from build123d import *

# Parameters (mm, degrees)
SKETCH1_R                        = 4.826
BOSS_EXTRUDE1_DEPTH              = 6.35
F_18_0_1695_DIAMETER_HOLE1_D     = 4.3053
F_18_0_1695_DIAMETER_HOLE1_DEPTH = 25.4
F_18_0_1695_DIAMETER_HOLE1_TIP   = 1.293442612
SKETCH4_R                        = 6.2992
SKETCH4_R_2                      = 6.35
CUT_EXTRUDE1_DEPTH               = 3.175
SKETCH5_R                        = 6.2992
CUT_EXTRUDE2_DEPTH               = 3.175
F_17_64_0_26563_DIAMETER_HOLE1_D = 6.747002


with BuildPart() as part:
    # Sketch1 → Boss-Extrude1 (new body)
    with BuildSketch(Plane(origin=(0, 0, 0), x_dir=(1, 0, 0), z_dir=(0, 1, 0))):
        with BuildLine():
            Line((0, 12.7), (114.3, 12.7))
            ThreePointArc((114.3, 12.7), (127, 0), (114.3, -12.7))
            Line((114.3, -12.7), (0, -12.7))
            ThreePointArc((0, -12.7), (-12.7, 0), (0, 12.7))
        make_face()
        Circle(SKETCH1_R, mode=Mode.SUBTRACT)
    extrude(amount=BOSS_EXTRUDE1_DEPTH)

    # #18 (0.1695) Diameter Hole1
    with Locations(Plane(origin=(0, 6.35, 0), x_dir=(1, 0, 0), z_dir=(0, 1, 0))):
        with Locations((-9.652, 0), (4.826, 8.358877197), (4.826, -8.358877197)):
            Hole(F_18_0_1695_DIAMETER_HOLE1_D / 2, depth=F_18_0_1695_DIAMETER_HOLE1_DEPTH)
            with Locations((0, 0, -(F_18_0_1695_DIAMETER_HOLE1_DEPTH + F_18_0_1695_DIAMETER_HOLE1_TIP / 2))):  # 118° drill point
                Cone(0, F_18_0_1695_DIAMETER_HOLE1_D / 2, F_18_0_1695_DIAMETER_HOLE1_TIP, mode=Mode.SUBTRACT)

    # Sketch4 → Cut-Extrude1 (cut)
    with BuildSketch(Plane(origin=(0, 6.35, 0), x_dir=(1, 0, 0), z_dir=(0, 1, 0))):
        with Locations((76.2, 0)):
            Circle(SKETCH4_R)
        with Locations((114.3, 0)):
            Circle(SKETCH4_R_2)
    extrude(amount=-CUT_EXTRUDE1_DEPTH, mode=Mode.SUBTRACT)

    # Sketch5 → Cut-Extrude2 (cut)
    with BuildSketch(Plane.XZ):
        with Locations((114.3, 0)):
            Circle(SKETCH5_R)
    extrude(amount=-CUT_EXTRUDE2_DEPTH, mode=Mode.SUBTRACT)

    # 17/64 (0.26563) Diameter Hole1 (through all)
    with Locations(Plane(origin=(0, 6.35, 0), x_dir=(1, 0, 0), z_dir=(0, 1, 0))):
        with Locations((76.2, 0), (114.3, 0)):
            Hole(F_17_64_0_26563_DIAMETER_HOLE1_D / 2)


solid = part.part
Work out the finished part from the listing and answer in its coordinate system (mm). A direction names the side the tool comes from. Round coordinates to 2 decimals unless told otherwise and drop trailing zeros. Write each loop counter-clockwise with the first axis right and the second up, starting at its lowest first coordinate (ties: lowest second). Pieces come first, ordered by that corner, then holes. Notation, with made-up numbers: (81.25, 46.25) -> (105.25, 46.25) arc R12 ccw to (105.25, 68.25) -> close; hole circle Ø9 at (6, 45). An arc over 180 degrees is marked (long way). Answer as CSV lines item,"result". Start each with the question number.
(1) A tool of negligible diameter and unlimited length cuts with its end or side. For faces 5 (the flat face through (58, 0, 0)), 6 (the flat face through (79, 3.175, 3)), from which of +Z, -Z, +X, -X, +Y, -Y can it reach the whole face along a straight path? Write none if from no direction.
(2) The mould has two halves that part along X. Classify faces 1 (the flat face through (58, 3, 12.7)), 2 (the cylindrical face through (71.2, 4.78, 3.83)), 3 (the cylindrical face through (-12.697, 3.131, 0.279)), 4 (the cylindrical face through (127, 3, 0)): +X half, -X half, draft (parallel to the pull), parting line (faces both ways), or undercut.
(3) Each of these flat-tipped pins is pushed along its axis until it touches: pin 1 (11 mm diameter, centred on x = 76.2, z = 0, fed in from +Y) (3 decimals); pin 2 (1 mm diameter, centred on x = 111, z = -9.5, fed in from -Y); pin 3 (3 mm diameter, centred on y = 3, z = 8.5, fed in from +X). Where does it stop, or does it pass through?
(4) Find the intervals of material crossed by probe 1 along Z at (x, y) = (114.3, 1.2); probe 2 along X at (y, z) = (4.75, 5.25); probe 3 along Z at (x, y) = (76.2, 2.05), in increasing order.
(5) The part is cut by section A-A, the plane z = 0. Give the number of separate pieces and of enclosed holes in the cut face, then the cut area to 3 significant figures.
(6) The part is cut by section B-B, the plane y = 5. Give the vertices of the cut face in (x, z), then the cut area to 3 significant figures.
Output values:
1,face 5,"+Z, -Z, +X, -X, -Y"
1,face 6,"+Y"
2,face 1,"draft"
2,face 2,"undercut"
2,face 3,"-X half"
2,face 4,"+X half"
3,pin 1,"stops at y = 3.175"
3,pin 2,"stops at y = 0"
3,pin 3,"stops at x = 124.9"
4,probe 1,"z = -12.7 to -6.3, 6.3 to 12.7"
4,probe 2,"x = -11.56 to 72.72, 79.68 to 110.73, 117.87 to 125.86"
4,probe 3,"z = -12.7 to -3.37, 3.37 to 12.7"
5,separate pieces,"5"
5,enclosed holes,"0"
5,area,"657 mm²"
6,outline,"(0, -12.7) -> (114.3, -12.7) arc R12.7 ccw to (114.3, 12.7) -> (0, 12.7) arc R12.7 ccw to start; hole circle Ø4.31 at (-9.65, 0); hole circle Ø9.65 at (0, 0); hole circle Ø4.31 at (4.83, -8.36); hole circle Ø4.31 at (4.83, 8.36); hole circle Ø12.6 at (76.2, 0); hole circle Ø12.7 at (114.3, 0)"
6,area,"3,040 mm²"
